The model under review builds one solid part; all positions refer to its coordinate system, in mm. A direction names the side the tool comes from. Round coordinates to 2 decimals unless told otherwise and drop trailing zeros. Order: outer loops, then holes, each group sorted by start corner. A loop starts at its lowest first (then second) coordinate and runs counter-clockwise, first axis right, second up.
```python
from build123d import *

# Parameters (mm, degrees)
SKETCH1_W           = 1237.47
SKETCH1_H           = 14
BOSS_EXTRUDE1_DEPTH = 133
LPATTERN3_COUNT     = 3
LPATTERN3_PITCH     = 300
CUT_EXTRUDE1_DEPTH  = 882.76981136
SKETCH3_W           = 91.937612072
SKETCH3_H           = 741.26
BOSS_EXTRUDE2_DEPTH = 10
SKETCH4_W           = 304.666106801
SKETCH4_H           = 263.446683033
CUT_EXTRUDE2_DEPTH  = 86
SKETCH5_R           = 8.65
CUT_EXTRUDE3_DEPTH  = 960.88018544
FILLET1_R           = 30
FILLET2_R           = 20
FILLET3_R           = 20
CUT_EXTRUDE4_DEPTH  = 960.88018544


with BuildPart() as part:
    # Sketch1 → Boss-Extrude1 (new body)
    with BuildSketch(Plane.XY):
        Rectangle(SKETCH1_W, SKETCH1_H)
    extrude(amount=BOSS_EXTRUDE1_DEPTH)


with BuildPart() as lpattern3_1:
    # LPattern3: pattern copy
    add(part.part.moved(Location(Vector(0, -1, 0) * (1 * LPATTERN3_PITCH))))


with BuildPart() as lpattern3_2:
    # LPattern3: pattern copy
    add(part.part.moved(Location(Vector(0, -1, 0) * (2 * LPATTERN3_PITCH))))


with BuildPart() as cut_extrude1_tool:
    # Sketch2 → Cut-Extrude1 (new, through all)
    with BuildSketch(Plane(origin=(0, 7, 0), x_dir=(1, 0, 0), z_dir=(0, 1, 0))):
        Polygon((-618.735, 0), (-618.735, -133), (-217.005, -133), (-217.005, -41.062387928), (-488.639842036, -15.767947981), (-489.975, 0), align=None)
        Polygon((217.005, -41.062387928), (488.639842036, -15.767947981), (489.975, 0), (618.735, 0), (618.735, -133), (217.005, -133), align=None)
    extrude(amount=-CUT_EXTRUDE1_DEPTH)


with BuildPart() as part_1:
    add(part.part)

    # Cut-Extrude1: cut by cut_extrude1_tool
    add(cut_extrude1_tool.part, mode=Mode.SUBTRACT)



with BuildPart() as lpattern3_1_1:
    add(lpattern3_1.part)

    # Cut-Extrude1: cut by cut_extrude1_tool
    add(cut_extrude1_tool.part, mode=Mode.SUBTRACT)


with BuildPart() as lpattern3_2_1:
    add(lpattern3_2.part)

    # Cut-Extrude1: cut by cut_extrude1_tool
    add(cut_extrude1_tool.part, mode=Mode.SUBTRACT)


with BuildPart() as part_2:
    add(part_1.part)

    add(lpattern3_1_1.part)  # Boss-Extrude2 merges LPattern3_1

    add(lpattern3_2_1.part)  # Boss-Extrude2 merges LPattern3_2
    # Sketch3 → Boss-Extrude2 (add)
    with BuildSketch(Plane.ZY.offset(217.005)):
        with Locations((87.031193964, -264.87)):
            Rectangle(SKETCH3_W, SKETCH3_H)
    boss_extrude2 = extrude(amount=-BOSS_EXTRUDE2_DEPTH)

    # Mirror1: Boss-Extrude2 across plane
    add(boss_extrude2.mirror(Plane(origin=(0, 0, 0), x_dir=(0, 0, 1), z_dir=(1, 0, 0))))

    # Sketch4 → Cut-Extrude2 (cut)
    with BuildSketch(Plane(origin=(0, 7, 0), x_dir=(1, 0, 0), z_dir=(0, 1, 0))):
        with Locations((-369.338053401, -91.037881314)):
            Rectangle(SKETCH4_W, SKETCH4_H)
        with Locations((369.338053401, -91.037881314)):
            Rectangle(SKETCH4_W, SKETCH4_H)
    extrude(amount=-CUT_EXTRUDE2_DEPTH, mode=Mode.SUBTRACT)

    # Sketch5 → Cut-Extrude3 (cut, through all)
    with BuildSketch(Plane.ZY.offset(217.005)):
        with Locations((66.922387928, 79.9)):
            Circle(SKETCH5_R)
        with BuildLine():
            Line((133, 75.48), (78.58674431, 102.979913133))
            ThreePointArc((78.58674431, 102.979913133), (53.374337442, 101.927027217), (41.062387928, 79.9))
            Line((41.062387928, 79.9), (30.442053439, 79.9))
            Line((30.442053439, 79.9), (30.442053439, 120.292255017))
            Line((30.442053439, 120.292255017), (142.138652578, 120.292255017))
            Line((142.138652578, 120.292255017), (142.138652578, 75.48))
            Line((142.138652578, 75.48), (133, 75.48))
        make_face()
    extrude(amount=-CUT_EXTRUDE3_DEPTH, mode=Mode.SUBTRACT)

    # Fillet1
    fillet1_edges = [part_2.edges().sort_by_distance(p)[0] for p in [
        (-217.005, 0, 0),
        (217.005, 0, 0),
    ]]
    fillet(fillet1_edges, radius=FILLET1_R)

    # Fillet2
    fillet2_edges = [part_2.edges().sort_by_distance(p)[0] for p in [
        (212.005, -635.5, 133),
        (212.005, -635.5, 41.062387928),
        (-212.005, -635.5, 41.062387928),
        (-212.005, -635.5, 133),
    ]]
    fillet(fillet2_edges, radius=FILLET2_R)

    # Fillet3
    # the kernel refuses this fillet: 20 mm, written as the material it takes off along each edge
    with BuildSketch(Plane(origin=(488.639842036, -251.216899092, 15.767947981), x_dir=(-0.995692394104561, 0, 0.0927181553005003), z_dir=(0, -1, 0))) as fillet3_piece_1:
        with BuildLine():
            CenterArc((16.713240363, 20), FILLET3_R, 192.778841583, 77.221158417)
            Line((-2.79138168, 15.576232492), (-3.181474121, 15.487757141))
            ThreePointArc((-3.181474121, 15.487757141), (-1.789418438, 7.717557206), (-0.393727599, -0.07055904))
            Line((-0.393727599, -0.07055904), (0, -0.4))
            Line((0, -0.4), (16.713240363, -0.4))
            Line((16.713240363, -0.4), (16.713240363, 0))
        make_face()
    extrude(amount=97.566201815, mode=Mode.SUBTRACT)
    with BuildSketch(Plane(origin=(488.639842036, -551.216899092, 15.767947981), x_dir=(0.08437350613868201, 0, -0.996434198259908), z_dir=(0, -1, 0))) as fillet3_piece_2:
        with BuildLine():
            CenterArc((16.738204459, -19.979111965), FILLET3_R, 92.618841583, 77.221158417)
            Line((-2.948175473, -16.451159984), (-3.341903071, -16.380600944))
            Line((-3.341903071, -16.380600944), (-0.393727599, 0.07055904))
            Line((-0.393727599, 0.07055904), (0, 0.4))
            ThreePointArc((0, 0.4), (7.912187282, 0.4), (15.806097965, 0.399582239))
            Line((15.806097965, 0.399582239), (15.824374563, 0))
        make_face()
    extrude(amount=97.566201815, mode=Mode.SUBTRACT)
    with BuildSketch(Plane(origin=(-488.639842036, -551.216899092, 15.767947981), x_dir=(0.995692394104561, 0, 0.0927181553005003), z_dir=(0, -1, 0)), Plane(origin=(-488.639842036, -251.216899092, 15.767947981), x_dir=(0.995692394104561, 0, 0.0927181553005003), z_dir=(0, -1, 0))) as fillet3_piece_3:
        with BuildLine():
            CenterArc((16.713240363, -20), FILLET3_R, 90, 77.221158417)
            Line((-2.79138168, -15.576232492), (-3.181474121, -15.487757141))
            ThreePointArc((-3.181474121, -15.487757141), (-1.789418438, -7.717557206), (-0.393727599, 0.07055904))
            Line((-0.393727599, 0.07055904), (0, 0.4))
            Line((0, 0.4), (16.713240363, 0.4))
            Line((16.713240363, 0.4), (16.713240363, 0))
        make_face()
    extrude(amount=97.566201815, mode=Mode.SUBTRACT)

    # Sketch6 → Cut-Extrude4 (cut, through all)
    with BuildSketch(Plane.ZY.offset(217.005)):
        with BuildLine():
            Line((109.261193964, -73.05), (109.261193964, -226.95))
            ThreePointArc((109.261193964, -226.95), (87.031193964, -249.18), (64.801193964, -226.95))
            Line((64.801193964, -226.95), (64.801193964, -73.05))
            ThreePointArc((64.801193964, -73.05), (87.031193964, -50.82), (109.261193964, -73.05))
        make_face()
        with BuildLine():
            Line((109.261193964, -526.95), (109.261193964, -373.05))
            ThreePointArc((109.261193964, -373.05), (87.031193964, -350.82), (64.801193964, -373.05))
            Line((64.801193964, -373.05), (64.801193964, -526.95))
            ThreePointArc((64.801193964, -526.95), (87.031193964, -549.18), (109.261193964, -526.95))
        make_face()
    extrude(amount=-CUT_EXTRUDE4_DEPTH, mode=Mode.SUBTRACT)


solid = part_2.part
```
(1) Consider section A-A (x = 138). Write out the cut boundary in (y, z), and give its area (3 significant figures).
Data:
outline: (-607, 0) - (-593, 0) - (-593, 133) - (-607, 133) - close; (-307, 0) - (-293, 0) - (-293, 133) - (-307, 133) - close; (-7, 0) - (7, 0) - (7, 133) - (-7, 133) - close
area: 5,590 mm2
(2) For faces 1 (the cylindrical face through (211.935, -50.825, 86.542)), 2 (the flat face through (207.005, -621, 86)), 3 (the cylindrical face through (207.98, 0.1, 8.55)), list the 3-axis set-ups (+Z, -Z, +X, -X, +Y, -Y) from which the entire face can be reached by the end or side of a thin tool; tool diameter is ignored.
Data:
face 1: +X, -X
face 2: +Z, -Z, -Y
face 3: -Z, +X, +Y
(3) Insertion check: pin 1 (15.5 mm diameter, centred on y = 79.9, z = 66.92, fed in from +X); pin 2 (3 mm diameter, centred on x = -210.5, y = -175.5, fed in from -Z); pin 3 (2 mm diameter, centred on y = -430, z = 52.5, fed in from +X) (3 decimals); pin 4 (8 mm diameter, centred on y = -39, z = 83.5, fed in from -X) (3 decimals). Each pin has a flat end and moves straight along its axis. Give the tip position at first contact, or say it passes through.
Data:
pin 1: passes through
pin 2: stops at z = 41.06
pin 3: stops at x = 217.005
pin 4: stops at x = -217.005
(4) Draft analysis for pull direction Y (two halves, no side actions). For faces 4 (the cylindrical face through (211.935, -350.825, 87.52)), 5 (the flat face through (1, -297, 133)), 6 (the flat face through (-212.08, 89.04, 106.17)), state which applies: pulls with the +Y half, pulls with the -Y half, needs draft (parallel to the pull), parting line crosses it, or undercut.
Data:
face 4: undercut
face 5: needs draft
face 6: pulls with the +Y half
(5) To check wall thickness, follow probe 1 along Y at (x, z) = (-3, 108.5); probe 2 along X at (y, z) = (-268, 111) (3 decimals); probe 3 along Y at (x, z) = (-292.5, 15.5). State the ranges of each line that lie inside material, in increasing order.
Data:
probe 1: y = -607 to -593, -307 to -293, -7 to 7
probe 2: x = -217.005 to -207.005, 207.005 to 217.005
probe 3: y = -607 to -593, -307 to -293
(6) Consider section B-B (y = -328.5). Write out the cut boundary in (x, z) (3 decimals), and give its area (3 significant figures).
Data:
outline: (-217.005, 41.062) - (-207.005, 41.062) - (-207.005, 133) - (-217.005, 133) - close; (207.005, 41.062) - (217.005, 41.062) - (217.005, 133) - (207.005, 133) - close
area: 1,840 mm2
(7) Consider section D-D (z = 89.5). State how many separate pieces and enclosed holes the cut face has, and give its area (3 significant figures).
Data:
separate pieces: 3
enclosed holes: 0
area: 24,100 mm2
(8) Consider section C-C (x = 352). Write out the cut boundary in (y, z).
Data:
outline: (-607, 0) - (-593, 0) - (-593, 28.49) - (-607, 28.49) - close; (-307, 0) - (-293, 0) - (-293, 28.49) - (-307, 28.49) - close
